```python
from build123d import *

# Parameters (mm, degrees)
SKETCH1_W           = 81
SKETCH1_H           = 20
BOSS_EXTRUDE2_DEPTH = 81
SKETCH2_R           = 9.5758
BOSS_EXTRUDE4_DEPTH = 10
SKETCH4_R           = 4.4958
CUT_EXTRUDE1_DEPTH  = 10


with BuildPart() as part:
    # Sketch1 → Boss-Extrude2 (new body)
    with BuildSketch(Plane(origin=(0, 0, 0), x_dir=(1, 0, 0), z_dir=(0, 1, 0))):
        Rectangle(SKETCH1_W, SKETCH1_H)
    extrude(amount=BOSS_EXTRUDE2_DEPTH)

    # Sketch2 → Boss-Extrude4 (add)
    with BuildSketch(Plane.XY.offset(10)):
        with Locations((-20.25, 40.5)):
            Circle(SKETCH2_R)
        with Locations((20.25, 40.5)):
            Circle(SKETCH2_R)
    extrude(amount=BOSS_EXTRUDE4_DEPTH)

    # Sketch4 → Cut-Extrude1 (cut)
    with BuildSketch(Plane.XY.offset(20)):
        with Locations((-20.510853934, 40.5563485)):
            Circle(SKETCH4_R)
        with Locations((20.060065936, 40.5563485)):
            Circle(SKETCH4_R)
    extrude(amount=-CUT_EXTRUDE1_DEPTH, mode=Mode.SUBTRACT)


solid = part.part
```
The listing builds one solid part. Answer for the finished solid, in the listing's coordinates (mm). A direction names the side the tool comes from. Coordinates: 2 decimals unless noted, no trailing zeros. Write each loop counter-clockwise with the first axis right and the second up, starting at its lowest first coordinate (ties: lowest second). Pieces come first, ordered by that corner, then holes. Notation, with made-up numbers: (33, 20.5) - (81, 20.5) arc R25 ccw to (81, 40.5) - close; hole circle Ø1 at (-17.75, -20). An arc over 180 degrees is marked (long way). Return JSON: item names as keys, results as strings. Group by question number.
Q1. Which of the six approach directions +Z, -Z, +X, -X, +Y, -Y give full straight-line access (tool end or side, diameter ignored) to faces 4 (the flat face through (-18, 36, 20)), 5 (the flat face through (-21, 41, 10))?
Q2. The part is cut by section C-C on y = 59. Write down the section's boundary in (x, z), and give its area (3 significant figures).
Q3. Flat-ended cylindrical pins translate along their axes: pin 1 Ø2.5 at (x, y) = (19.5, 41.5) entering from +Z; pin 2 Ø4 at (x, z) = (14.5, 12.5) entering from -Y. Find the tip coordinate at first contact, or state that the pin passes through.
Q4. The part is cut by section D-D on x = 20.25. Write down the section's boundary in (y, z), and give its area (3 significant figures).
Q5. The part is cut by section B-B on z = 18.25. Write down the section's boundary in (x, y).
Q6. Find the intervals of material crossed by line 1 along Z through (x, y) = (21, 53); line 2 along Y through (x, z) = (12, 15.5), in increasing order. Write a range as [from, to].
Q7. The part is cut by section A-A on x = -28.5. Write down the section's boundary in (y, z).
Q8. For a pull along X with two mould halves and no side action, classify faces 1 (the flat face through (-40.5, 40, 0)), 2 (the flat face through (-1, 40, -10)), 3 (the flat face through (20, 41, 10)) as +X half, -X half, draft (parallel to the pull), parting line (faces both ways), or undercut.
Evaluation:
{
 "1": {"face 4": "+Z, +X, -X, +Y, -Y", "face 5": "+Z"},
 "2": {"outline": "(-40.5, -10) - (40.5, -10) - (40.5, 10) - (-40.5, 10) - close", "area": "1,620 mm2"},
 "3": {"pin 1": "stops at z = 10", "pin 2": "stops at y = 31.69"},
 "4": {"outline": "(0, -10) - (81, -10) - (81, 10) - (50.08, 10) - (50.08, 20) - (45.05, 20) - (45.05, 10) - (36.06, 10) - (36.06, 20) - (30.92, 20) - (30.92, 10) - (0, 10) - close", "area": "1,720 mm2"},
 "5": {"outline": "circle Ø19.15 at (-20.25, 40.5); circle Ø19.15 at (20.25, 40.5); hole circle Ø8.99 at (-20.51, 40.56); hole circle Ø8.99 at (20.06, 40.56)"},
 "6": {"line 1": "z = [-10, 10]", "line 2": "y = [35.64, 45.36]"},
 "7": {"outline": "(0, -10) - (81, -10) - (81, 10) - (45.36, 10) - (45.36, 20) - (35.64, 20) - (35.64, 10) - (0, 10) - close"},
 "8": {"face 1": "-X half", "face 2": "draft", "face 3": "undercut"}
}
